Can you work these out from the model? Positions are in its coordinate system, mm. Face numbers are marked on the shaded views. A direction names the side the tool comes from. Round coordinates to 2 decimals unless told otherwise and drop trailing zeros. Order: outer loops, then holes, each group sorted by start corner. A loop starts at its lowest first (then second) coordinate and runs counter-clockwise, first axis right, second up.
from build123d import *

# Parameters (mm, degrees)
PAD007_DEPTH = 2
SKETCH012_R  = 1.375
PAD004_DEPTH = 6


with BuildPart() as slotscrew:
    # Sketch020 → Pad007 (new body)
    with BuildSketch(Plane.XZ):
        with BuildLine():
            ThreePointArc((8.9, 35), (5.9, 38), (2.9, 35))
            Line((2.9, 35), (2.9, 13))
            ThreePointArc((2.9, 13), (5.9, 10), (8.9, 13))
            Line((8.9, 13), (8.9, 35))
        make_face()
    extrude(amount=PAD007_DEPTH)


with BuildPart() as slotscrew_1:
    # Body009 placement: moved
    add(slotscrew.part.moved(Location((-0.028, 0.002, -39.747))))


with BuildPart() as base:
    # Sketch012 → Pad004 (new body)
    with BuildSketch(Plane.XZ):
        with BuildLine():
            Line((-4, 0), (10, 0))
            Line((10, 0), (10, -30.2))
            ThreePointArc((8.2, -32), (9.472792, -31.472792), (10, -30.2))
            Line((8.2, -32), (-2.2, -32))
            ThreePointArc((-4, -30.2), (-3.472792, -31.472792), (-2.2, -32))
            Line((-4, -30.2), (-4, 0))
        make_face()
        with Locations((-1.9, -15.9)):
            Circle(SKETCH012_R, mode=Mode.SUBTRACT)
        with BuildLine():
            ThreePointArc((4.4, -26.9), (5.9, -28.4), (7.4, -26.9))
            Line((7.4, -26.9), (7.4, -4.9))
            ThreePointArc((7.4, -4.9), (5.9, -3.4), (4.4, -4.9))
            Line((4.4, -4.9), (4.4, -26.9))
        make_face(mode=Mode.SUBTRACT)
    extrude(amount=PAD004_DEPTH)

    # Cut044: cut slotscrew
    add(slotscrew_1.part, mode=Mode.SUBTRACT)


with BuildPart() as base_1:
    # Cut044 placement: moved
    add(base.part.moved(Location((0, 5.988, 0))))


solid = base_1.part
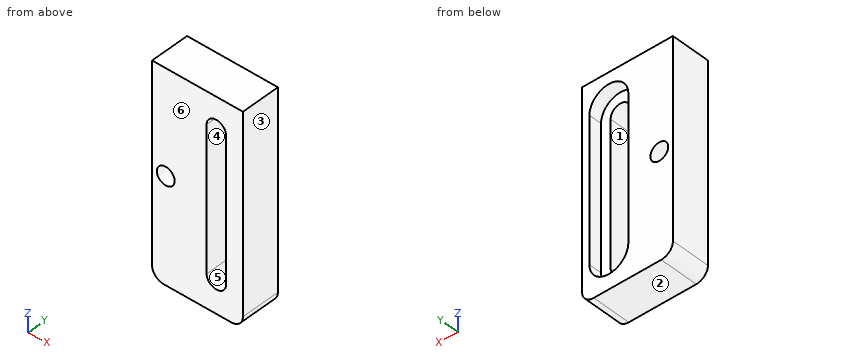
(1) On a 3-axis mill with a long thin cutter (end or side, diameter ignored), from which of +Z, -Z, +X, -X, +Y, -Y can I reach the whole of each face in a straight line? I mean the marked faces 5 and 6. Say none if no direction works.
(2) If we mould it in two halves opening along Z, with no side actions, what happens to the marked faces 1, 2, 3 and 4? For each: pulls with the +Z half, pulls with the -Z half, needs draft (parallel to the pull), parting line crosses it, or undercut.
(3) Please list where these lines run through material, in increasing order: probe 1 along X at (y, z) = (3.25, -22.5); probe 2 along Z at (x, y) = (-1.9, 3.05) (3 decimals); probe 3 along X at (y, z) = (3.3, -17) (3 decimals).
(4) I want a section at D-D, the plane x = 3.5. List the corners of the cut face in (y, z) for me.
(5) I want a section at C-C, the plane y = 2.7. List the corners of the cut face in (x, z) for me (3 decimals).
(6) I want a section at B-B, the plane z = -18. List the corners of the cut face in (x, y) for me, plus the area to 3 significant figures.
(7) I'm going to push flat-ended pins straight in: pin 1 Ø3 at (x, z) = (6, -17) entering from +Y; pin 2 Ø2.5 at (x, z) = (-1.9, -15.9) entering from -Y. Where does each tip first touch, or does it pass through?
(8) I want a section at A-A, the plane x = -1.9. List the corners of the cut face in (y, z) for me (3 decimals), plus the area to 4 significant figures.
Ans:
1. face 5: +Y, -Y
1. face 6: +Z, -Z, +X, -X, -Y
2. face 1: undercut
2. face 2: pulls with the -Z half
2. face 3: needs draft
2. face 4: undercut
3. probe 1: x = -4 to 4.4, 7.4 to 10
3. probe 2: z = -32 to -17.275, -14.525 to 0
3. probe 3: x = -4 to -2.725, -1.075 to 4.4, 7.4 to 10
4. outline: (-0.01, -32) - (5.99, -32) - (5.99, -28.58) - (3.99, -28.58) - (3.99, -2.91) - (5.99, -2.91) - (5.99, 0) - (-0.01, 0) - close
5. outline: (-4, -30.2) arc R1.8 ccw to (-2.2, -32) - (8.2, -32) arc R1.8 ccw to (10, -30.2) - (10, 0) - (-4, 0) - close; hole circle Ø2.75 at (-1.9, -15.9); hole (4.4, -26.9) arc R1.5 ccw to (7.4, -26.9) - (7.4, -4.9) arc R1.5 ccw to (4.4, -4.9) - close
6. outline: (-4, -0.01) - (4.4, -0.01) - (4.4, 3.99) - (2.87, 3.99) - (2.87, 5.99) - (-4, 5.99) - close; (7.4, -0.01) - (10, -0.01) - (10, 5.99) - (8.87, 5.99) - (8.87, 3.99) - (7.4, 3.99) - close
6. area: 60.0 mm2
7. pin 1: stops at y = 3.99
7. pin 2: passes through
8. outline: (-0.012, -32) - (5.988, -32) - (5.988, -17.275) - (-0.012, -17.275) - close; (-0.012, -14.525) - (5.988, -14.525) - (5.988, 0) - (-0.012, 0) - close
8. area: 175.5 mm2
